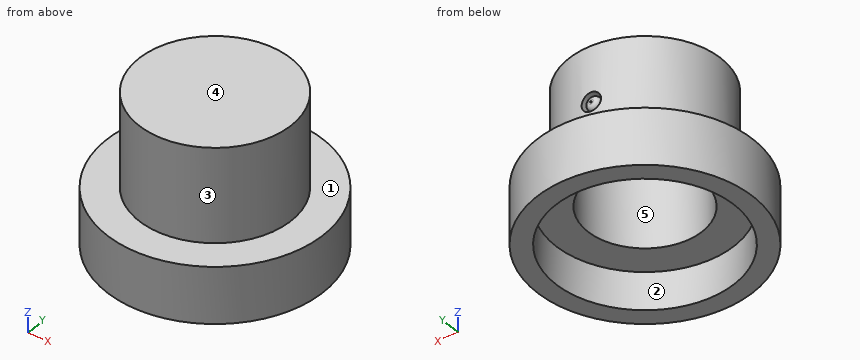
```python
from build123d import *

# Parameters (mm, degrees)
F0_R      = 11.5
F1_DEPTH  = 6
F2_T      = -2
F3_R      = 8.0805542871
F4_DEPTH  = 10
F5_T      = 2
F7_R      = 1
F8_DEPTH  = 7
F9_R      = 0.75
F10_DEPTH = 1
F11_R     = 0.5
F12_R     = 0.0887059055
F13_DEPTH = 7


# Not quite as in the source:
# - a shell that OpenCascade refuses in one call is made with other operations: the cavity is built on its own and cut out


with BuildPart() as f1:
    # F0 (on Top) → F1 (new body)
    with BuildSketch(Plane.XY):
        with Locations((-24.4241058826, 15.6410522759)):
            Circle(F0_R)
    extrude(amount=F1_DEPTH)

    # F2
    f2_openings = [f1.faces().sort_by_distance(p)[0] for p in [
        (-24.424106, 15.641052, 0),
    ]]
    offset(amount=F2_T, openings=f2_openings)

    # F3 (on face) → F4 (join)
    with BuildSketch(Plane.XY.offset(6)):
        with Locations((-24.4241058826, 15.6410522759)):
            Circle(F3_R)
    extrude(amount=F4_DEPTH)

    # F5: shell of thickness 2, made by hand


with BuildPart() as f5_core1:
    # F5_t2: copy of F1
    add(f1.part)

    # the walls: a layer under each face that stays
    f5_faces = [f5_core1.faces().sort_by_distance(p)[0] for p in [
        (-35.9241058826, 15.6410522759, 3),
        (-32.0907725493, 7.9743856092, 0),
        (-32.0907725493, 7.9743856092, 6),
        (-33.9241058826, 15.6410522759, 2),
        (-32.5046601698, 15.6410522759, 11),
        (-24.4241058826, 15.6410522759, 16),
    ]]
    thicken(f5_faces, amount=-F5_T, mode=Mode.SUBTRACT)

    # F5_s3 → F5_t4 (revolve, cut)
    with BuildSketch(Plane.XZ.offset(-15.6410522759)):
        Polygon((-16.3235515955, 6.02), (-16.3435515955, 4), (-18.3435515955, 4), (-18.3435515955, 6), align=None)
    revolve(axis=Axis((-24.4241058826, 15.6410522759, 6), (0, 0, 1)), mode=Mode.SUBTRACT)


with BuildPart() as f1_1:
    add(f1.part)

    # what is left inside the walls is the cavity
    f5_cavity = [f5_core1.part.solids().sort_by_distance(p)[0] for p in [
        (-30.48466, 15.641052, 11.333333),
    ]]
    add(f5_cavity, mode=Mode.SUBTRACT)

    # F7 (on offset) → F8 (cut)
    with BuildSketch(Plane.XZ.offset(-29.7)):
        with Locations((-24.9341819435, 10.1343514398)):
            Circle(F7_R)
    extrude(amount=F8_DEPTH, mode=Mode.SUBTRACT)

    # F9 (on face) → F10 (join)
    with BuildSketch(Plane(origin=(0, 22.7, 0), x_dir=(-1, 0, 0), z_dir=(0, 1, 0))):
        with Locations((24.9341819435, 10.1343514398)):
            Circle(F9_R)
    extrude(amount=F10_DEPTH)

    # F11
    f11_edges = [f1_1.edges().sort_by_distance(p)[0] for p in [
        (-24.184182, 23.7, 10.134351),
    ]]
    fillet(f11_edges, radius=F11_R)

    # F12 (on face) → F13 (cut)
    with BuildSketch(Plane(origin=(0, 23.7, 0), x_dir=(-1, 0, 0), z_dir=(0, 1, 0))):
        with Locations((24.9341819435, 10.1343514398)):
            Circle(F12_R)
    extrude(amount=-F13_DEPTH, mode=Mode.SUBTRACT)


solid = f1_1.part
```
Source: CAD feature listing. Evaluate the final solid. Frame: model axes, mm. Face numbers are marked on the shaded views. A direction names the side the tool comes from. Round coordinates to 2 decimals unless told otherwise and drop trailing zeros. Write each loop counter-clockwise with the first axis right and the second up, starting at its lowest first coordinate (ties: lowest second). Pieces come first, ordered by that corner, then holes. Notation, with made-up numbers: M 60,82 L 76,82 A18 cw 76,99 Z; hole C 39.25,57 d11. An arc over 180 degrees is marked long. Use CSV: the item, a comma, the result in double quotes. Start each with the question number.
Q1. Line query: line 1 (X direction, y = 19, z = 2); line 2 (X direction, y = 12.5, z = 6.5); line 3 (Y direction, x = -23.75, z = 7.5). Output: solid intervals per line, ascending. Write a range as from..to.
Q2. Cut plane B-B on x = -22.5. Output: boundary loops of the cut face in (y, z), plus the area to 3 significant figures.
Q3. Cut plane A-A on y = 17.75. Output: boundary loops of the cut face in (x, z), plus the area to 3 significant figures.
Q4. First-contact query: P1, Ø1.5, axis at x = -22, z = 12.5, coming from the -Y side; P2, Ø1.6, axis at x = -24.93, z = 10.13, coming from the -Y side; P3, Ø13.5, axis at x = -25, y = 17.5, coming from the -Z side; P4, Ø6, axis at y = 15, z = 6, coming from the -X side. Flat tips, straight axial feed; report the tip coordinate or a pass-through.
Q5. Pull-direction query (X, two-part tool) for the marked faces 1, 2 and 3; classes: +X half, -X half, draft (parallel to the pull), parting line (faces both ways), or undercut.
Q6. Cut plane C-C on z = 8.5. Output: boundary loops of the cut face in (x, y), plus the area to 3 significant figures.
Q7. Access query for the marked faces 4 and 5. Directions: +Z, -Z, +X, -X, +Y, -Y. A direction counts if a zero-diameter tool reaches every point of the face in a straight line with its end or side. Return the directions, or none.
Q8. Cut plane D-D on y = 7. Output: boundary loops of the cut face in (x, z), plus the area to 3 significant figures.
Results found:
1,line 1,"-35.42..-33.31, -15.54..-13.43"
1,line 2,"-31.87..-29.63, -19.22..-16.98"
1,line 3,"7.59..9.6, 21.68..23.69"
2,outline,"M 4.3,0 L 6.34,0 L 6.34,4 L 9.87,4 L 9.87,14 L 21.41,14 L 21.41,4 L 24.94,4 L 24.94,0 L 26.98,0 L 26.98,6 L 23.49,6 L 23.49,16 L 7.79,16 L 7.79,6 L 4.3,6 Z"
2,area,"103 mm^2"
3,outline,"M -35.73,0 L -33.69,0 L -33.69,4 L -30.13,4 L -30.13,14 L -18.72,14 L -18.72,4 L -15.16,4 L -15.16,0 L -13.12,0 L -13.12,6 L -16.62,6 L -16.62,16 L -32.22,16 L -32.22,6 L -35.73,6 Z"
3,area,"104 mm^2"
4,P1,"y = 7.74"
4,P2,"y = 7.56"
4,P3,"z = 4"
4,P4,"x = -35.92"
5,face 1,"draft"
5,face 2,"undercut"
5,face 3,"parting line"
6,outline,"C -24.42,15.64 d16.16; hole C -24.42,15.64 d12.16"
6,area,"89.0 mm^2"
7,face 4,"+Z, +X, -X, +Y, -Y"
7,face 5,"-Z"
8,outline,"M -32.01,0 L -28.37,0 L -28.37,4 L -20.48,4 L -20.48,0 L -16.84,0 L -16.84,6 L -32.01,6 Z"
8,area,"59.5 mm^2"
